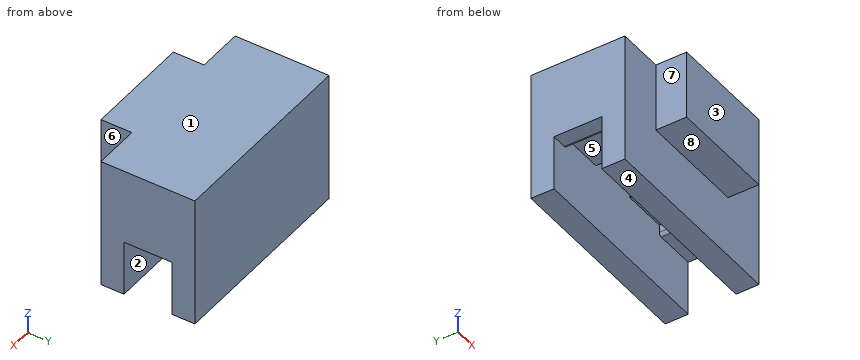
```python
from build123d import *

# Parameters (mm, degrees)
F0_W     = 13
F0_H     = 1.5
F1_DEPTH = 3.6
F2_W     = 13
F2_H     = 6.1
F3_DEPTH = 4.91
F4_W     = 9
F4_H     = 3.1
F5_DEPTH = 0.7
F6_W     = 3.3
F6_H     = 3.1
F7_DEPTH = 0.7
F8_W     = 7
F8_H     = 4.5
F9_DEPTH = 2
F10_R    = 0.2


with BuildPart() as f1:
    # F0 (on Top) → F1 (new body)
    with BuildSketch(Plane.XY):
        with Locations((0, 2.3)):
            Rectangle(F0_W, F0_H)
        with Locations((0, -2.3)):
            Rectangle(F0_W, F0_H)
    extrude(amount=-F1_DEPTH)

    # F2 (on Top) → F3 (join)
    with BuildSketch(Plane.XY):
        Rectangle(F2_W, F2_H)
    extrude(amount=F3_DEPTH)

    # F4 (on face) → F5 (cut)
    with BuildSketch(Plane(origin=(0, 0, 0), x_dir=(1, 0, 0), z_dir=(0, 0, -1))):
        with Locations((-0.8, 0)):
            Rectangle(F4_W, F4_H)
    extrude(amount=-F5_DEPTH, mode=Mode.SUBTRACT)

    # F6 (on face) → F7 (cut)
    with BuildSketch(Plane(origin=(0, 0, 0.7), x_dir=(1, 0, 0), z_dir=(0, 0, -1))):
        with Locations((-0.8, 0)):
            Rectangle(F6_W, F6_H)
    extrude(amount=-F7_DEPTH, mode=Mode.SUBTRACT)

    # F8 (on face) → F9 (join)
    with BuildSketch(Plane.XZ.offset(3.05)):
        with Locations((0, 2.66)):
            Rectangle(F8_W, F8_H)
    extrude(amount=F9_DEPTH)

    # F10
    f10_edges = [f1.edges().sort_by_distance(p)[0] for p in [
        (-5.3, 0, 0),
        (3.7, 0, 0),
    ]]
    fillet(f10_edges, radius=F10_R)


solid = f1.part
```
Design review of the part built by this model. Coordinates are the model's own, in mm. Face numbers are marked on the shaded views. A direction names the side the tool comes from. Give positions to 0.01 mm unless a question says otherwise; leave off trailing zeros. Loops run counter-clockwise (first coordinate to the right, second up) from the corner with the lowest first, then second, coordinate; pieces in that order, holes last. Notation, with made-up numbers: (78, -27) -> (83, -27) arc R22 cw to (83, 7) -> close; hole circle Ø5 at (-14.75, 37.5). An arc over 180 degrees is marked (long way). One line per item, written item: value.
Q1. We need section B-B on z = -1.25. Give the boundary of the cut face in (x, y), and give its area (3 significant figures).
Numbers:
outline: (-6.5, -3.05) -> (6.5, -3.05) -> (6.5, -1.55) -> (-6.5, -1.55) -> close; (-6.5, 1.55) -> (6.5, 1.55) -> (6.5, 3.05) -> (-6.5, 3.05) -> close
area: 39.0 mm^2
Q2. We need section D-D on y = -0.5. Give the boundary of the cut face in (x, z).
Numbers:
outline: (-6.5, 0) -> (-5.5, 0) arc R0.2 ccw to (-5.3, 0.2) -> (-5.3, 0.7) -> (-2.45, 0.7) -> (-2.45, 1.4) -> (0.85, 1.4) -> (0.85, 0.7) -> (3.7, 0.7) -> (3.7, 0.2) arc R0.2 ccw to (3.9, 0) -> (6.5, 0) -> (6.5, 4.91) -> (-6.5, 4.91) -> close
Q3. We need section C-C on x = -4.75. Give the boundary of the cut face in (y, z).
Numbers:
outline: (-3.05, -3.6) -> (-1.55, -3.6) -> (-1.55, 0.7) -> (1.55, 0.7) -> (1.55, -3.6) -> (3.05, -3.6) -> (3.05, 4.91) -> (-3.05, 4.91) -> close
Q4. Draft analysis for pull direction Y (two halves, no side actions). For the marked faces 1, 2 and 3, state which applies: pulls with the +Y half, pulls with the -Y half, needs draft (parallel to the pull), parting line crosses it, or undercut.
Numbers:
face 1: needs draft
face 2: undercut
face 3: pulls with the -Y half
Q5. For L1, parallel to Y at x = 5, z = -2.75; L2, parallel to X at y = 0, z = 0.75, list the stretches that pass through material, from the lowest coordinate up.
Numbers:
L1: y = -3.05 to -1.55, 1.55 to 3.05
L2: x = -6.5 to -2.45, 0.85 to 6.5
Q6. We need section A-A on z = 1. Give the boundary of the cut face in (x, y).
Numbers:
outline: (-6.5, -3.05) -> (-3.5, -3.05) -> (-3.5, -5.05) -> (3.5, -5.05) -> (3.5, -3.05) -> (6.5, -3.05) -> (6.5, 3.05) -> (-6.5, 3.05) -> close; hole (-2.45, -1.55) -> (0.85, -1.55) -> (0.85, 1.55) -> (-2.45, 1.55) -> close
Q7. Machinability: for the marked faces 4, 5, 6, 7 and 8, which of the approach directions +Z, -Z, +X, -X, +Y, -Y give a long, thin tool a straight path to every point of the face, cutting with its end or side? Answer none if there is none.
Numbers:
face 4: -Z, +X, -X, +Y, -Y
face 5: -Z
face 6: +Z, -Z, +X, -Y
face 7: +Z, -Z, -X, -Y
face 8: -Z, +X, -X, -Y
Q8. For pin 1 Ø1 at (x, y) = (-1.5, -4) entering from -Z; pin 2 Ø0.5 at (x, y) = (-6, -0.5) entering from -Z; pin 3 Ø1 at (y, z) = (-4, 3.5) entering from +X, all flat-tipped, find the tip position at first contact; note any pin that passes through.
Numbers:
pin 1: stops at z = 0.41
pin 2: stops at z = 0
pin 3: stops at x = 3.5
